```python
from build123d import *

# Parameters (mm, degrees)
SKETCH1_W           = 54
SKETCH1_H           = 25
BOSS_EXTRUDE1_DEPTH = 10
SKETCH2_R           = 1.25
SKETCH2_R_2         = 4.5
SKETCH2_R_3         = 1.541692257
SKETCH2_R_4         = 1.457345452
SKETCH2_W           = 17
SKETCH2_H           = 15
CUT_EXTRUDE1_DEPTH  = 10


with BuildPart() as part:
    # Sketch1 → Boss-Extrude1 (new body)
    with BuildSketch(Plane(origin=(0, 0, 0), x_dir=(1, 0, 0), z_dir=(0, 1, 0))):
        with Locations((27, 12.5)):
            Rectangle(SKETCH1_W, SKETCH1_H)
    extrude(amount=BOSS_EXTRUDE1_DEPTH)

    # Sketch2 → Cut-Extrude1 (cut)
    with BuildSketch(Plane(origin=(0, 10, 0), x_dir=(1, 0, 0), z_dir=(0, 1, 0))):
        with Locations(Location((49, 13.5, 0), (0, 0, 270))):
            Circle(SKETCH2_R)
        with Locations(Location((5, 13.5, 0), (0, 0, 270))):
            Circle(SKETCH2_R)
        with Locations(Location((22, 10.5, 0), (0, 0, 270))):
            Circle(SKETCH2_R_2)
        with Locations(Location((14, 13, 0), (0, 0, 270))):
            Circle(SKETCH2_R_3)
        with Locations(Location((14, 8, 0), (0, 0, 270))):
            Circle(SKETCH2_R_4)
        with Locations((36.5, 12.5)):
            Rectangle(SKETCH2_W, SKETCH2_H)
    extrude(amount=-CUT_EXTRUDE1_DEPTH, mode=Mode.SUBTRACT)


solid = part.part
```
Verification items for the finished model (mm, model axes). A direction names the side the tool comes from. Coordinates: 2 decimals unless noted, no trailing zeros. Write each loop counter-clockwise with the first axis right and the second up, starting at its lowest first coordinate (ties: lowest second). Pieces come first, ordered by that corner, then holes. Notation, with made-up numbers: (74.5, 87.5) - (110.5, 87.5) arc R22 ccw to (110.5, 106.5) - close; hole circle Ø5 at (41, 28.5). An arc over 180 degrees is marked (long way). One line per question, with ' | ' between items. Start each with the question number.
1. Draft check along X on faces 1 (the cylindrical face through (12.495, 5.07, -13.334)), 2 (the flat face through (27, 5, 0)), 3 (the flat face through (54, 5, -12)). Enter one of: released by +X, released by -X, zero draft, split by the parting line, or undercut.
2. Section check B-B (x = 22). Enter the section's corners in (y, z).
3. Access from +Z, -Z, +X, -X, +Y, -Y to the whole of each face (thin tool, end or side, straight path). Record for faces 4 (the flat face through (45, 5, -12)), 5 (the flat face through (27, 0, -13)).
4. Section check D-D (z = -10.5). Enter the section's corners in (x, y), plus the area to 3 significant figures.
5. Section check A-A (x = 14). Enter the section's corners in (y, z), plus the area to 3 significant figures.
6. Gauge pin test, flat end, axial feed: P1, Ø2, axis at x = 49, z = -13.5, coming from the +Y side. Record the tip position at first contact, or that the pin passes through.
7. Material ranges on line 1 along X through (y, z) = (4.5, -10.5); line 2 along X through (y, z) = (5, -16.25); line 3 along X through (y, z) = (8.5, -7.5), recorded low to high.
8. Section check C-C (z = -14). Enter the section's corners in (x, y).
Computed values:
1) face 1: undercut | face 2: zero draft | face 3: released by +X
2) outline: (0, -25) - (10, -25) - (10, -15) - (0, -15) - close; (0, -6) - (10, -6) - (10, 0) - (0, 0) - close
3) face 4: +Y, -Y | face 5: +Z, -Z, +X, -X, -Y
4) outline: (0, 0) - (17.5, 0) - (17.5, 10) - (0, 10) - close; (26.5, 0) - (28, 0) - (28, 10) - (26.5, 10) - close; (45, 0) - (54, 0) - (54, 10) - (45, 10) - close | area: 280 mm²
5) outline: (0, -25) - (10, -25) - (10, -14.54) - (0, -14.54) - close; (0, -11.46) - (10, -11.46) - (10, -9.46) - (0, -9.46) - close; (0, -6.54) - (10, -6.54) - (10, 0) - (0, 0) - close | area: 190 mm²
6) P1: through
7) line 1: 0 to 17.5, 26.5 to 28, 45 to 54 | line 2: 0 to 28, 45 to 54 | line 3: 0 to 12.63, 15.37 to 18.65, 25.35 to 28, 45 to 54
8) outline: (0, 0) - (3.85, 0) - (3.85, 10) - (0, 10) - close; (6.15, 0) - (12.83, 0) - (12.83, 10) - (6.15, 10) - close; (15.17, 0) - (19.17, 0) - (19.17, 10) - (15.17, 10) - close; (24.83, 0) - (28, 0) - (28, 10) - (24.83, 10) - close; (45, 0) - (47.85, 0) - (47.85, 10) - (45, 10) - close; (50.15, 0) - (54, 0) - (54, 10) - (50.15, 10) - close
